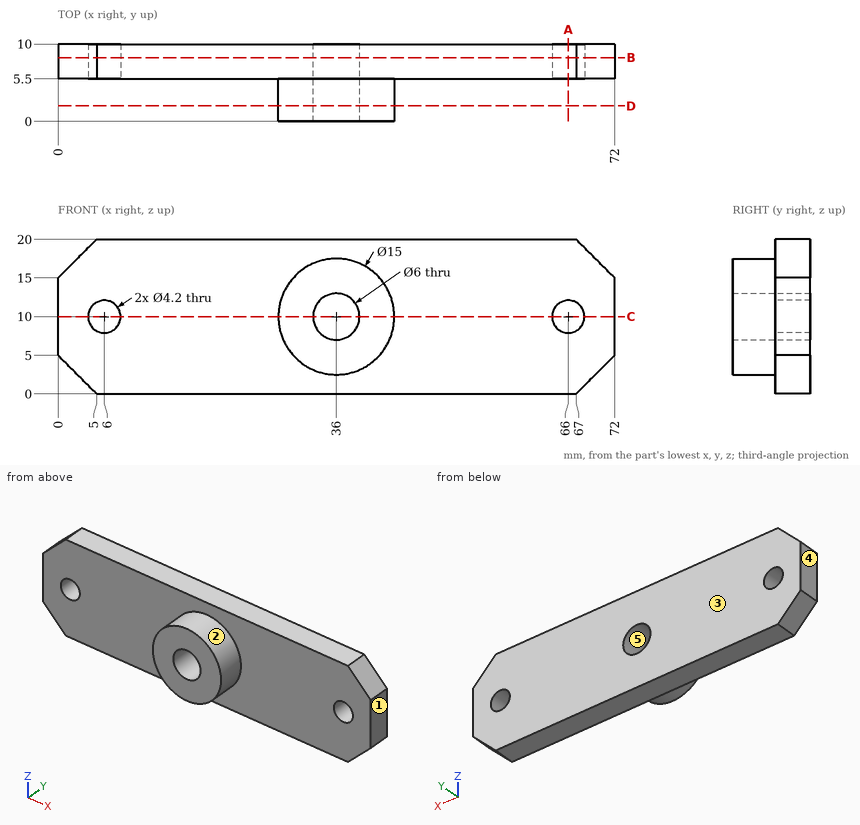
Input: dimensioned drawing with shaded views. Units: mm. Origin: part minimum x, y, z. A direction names the side the tool comes from. Give positions to 0.01 mm unless a question says otherwise; leave off trailing zeros. Write each loop counter-clockwise with the first axis right and the second up, starting at its lowest first coordinate (ties: lowest second). Pieces come first, ordered by that corner, then holes. Notation, with made-up numbers: (60.5, -33) - (113.5, -33) arc R13 cw to (113.5, -12) - close; hole circle Ø3 at (8.5, 57). An arc over 180 degrees is marked (long way). One line per item, written item: value. Start each with the question number.
Q1. Section query D-D, the plane y = 2. Return the cut outline in (x, z), then the cut area to 3 significant figures.
Q2. Section query A-A, the plane x = 66. Return the cut outline in (y, z), then the cut area to 3 significant figures.
Q3. First-contact query: pin 1 Ø2 at (x, z) = (38, 14.5) entering from -Y; pin 2 Ø3.5 at (x, z) = (36, 10) entering from -Y; pin 3 Ø5 at (x, z) = (6, 10) entering from -Y. Flat tips, straight axial feed; report the tip coordinate or a pass-through.
Q4. Material intervals for probe 1 along Z at (x, y) = (6, 6.5); probe 2 along Z at (x, y) = (36, 4.5); probe 3 along Y at (x, z) = (55.5, 13.25), sorted ascending. Write a range as from..to.
Q5. Set-up query: the marked faces 1 and 2. Return all of +Z, -Z, +X, -X, +Y, -Y with unobstructed straight access to the full face (end or side cutting, diameter ignored); none if empty.
Q6. Section query B-B, the plane y = 8.25. Return the cut outline in (x, z).
Q7. Draft query along X for the marked faces 3, 4 and 5. Return one class per face: +X half, -X half, draft (parallel to the pull), parting line (faces both ways), or undercut.
Q8. Section query C-C, the plane z = 10. Return the cut outline in (x, y), then the cut area to 3 significant figures.
Answer:
1. outline: circle Ø15 at (36, 10); hole circle Ø6 at (36, 10)
1. area: 148 mm2
2. outline: (5.5, 0) - (10, 0) - (10, 7.9) - (5.5, 7.9) - close; (5.5, 12.1) - (10, 12.1) - (10, 20) - (5.5, 20) - close
2. area: 71.1 mm2
3. pin 1: stops at y = 0
3. pin 2: passes through
3. pin 3: stops at y = 5.5
4. probe 1: z = 0..7.9, 12.1..20
4. probe 2: z = 2.5..7, 13..17.5
4. probe 3: y = 5.5..10
5. face 1: +Z, -Z, +X, +Y, -Y
5. face 2: -Y
6. outline: (0, 5) - (5, 0) - (67, 0) - (72, 5) - (72, 15) - (67, 20) - (5, 20) - (0, 15) - close; hole circle Ø4.2 at (6, 10); hole circle Ø6 at (36, 10); hole circle Ø4.2 at (66, 10)
7. face 3: draft
7. face 4: -X half
7. face 5: undercut
8. outline: (0, 5.5) - (3.9, 5.5) - (3.9, 10) - (0, 10) - close; (8.1, 5.5) - (28.5, 5.5) - (28.5, 0) - (33, 0) - (33, 10) - (8.1, 10) - close; (39, 0) - (43.5, 0) - (43.5, 5.5) - (63.9, 5.5) - (63.9, 10) - (39, 10) - close; (68.1, 5.5) - (72, 5.5) - (72, 10) - (68.1, 10) - close
8. area: 309 mm2
